Autodesk Inventor part; units mm, degrees
ref_plane "YZ Plane" through (0, 0, 0) normal (1, 0, 0) x (0, 1, 0)
ref_plane "XZ Plane" through (0, 0, 0) normal (0, 1, 0) x (-1, 0, 0)
ref_plane "XY Plane" through (0, 0, 0) normal (0, 0, 1) x (1, 0, 0)
sketch "Sketch15" plane through (0, 0, 0) normal (1, 0, 0) x (0, 1, 0)
  line L0 (0, 0) -> (50.8, 0)
  line L1 (50.8, 0) -> (50.8, 25.4)
  line L2 (50.8, 25.4) -> (0, 25.4)
  line L3 (0, 25.4) -> (0, 0)
  line L4 (48.26, 22.86) -> (2.54, 22.86)
  line L5 (2.54, 22.86) -> (2.54, 2.54)
  line L6 (2.54, 2.54) -> (48.26, 2.54)
  line L7 (48.26, 2.54) -> (48.26, 22.86)
  dimension "d46" = 25.4
  dimension "d47" = 50.8
  dimension "d48" = 2.54
  dimension "d49" = 2.54
  dimension "d50" = 2.54
  dimension "d51" = 2.54
extrude "Extrusion12" add sketch "Sketch15" along normal blind 76.2
sketch "Sketch17" plane through (0, 0, 0) normal (0, 0, -1) x (-1, 0, 0)
  line L0 (0, 2.54) -> (-76.2, 2.54)
  line L1 (0, 48.26) -> (-76.2, 48.26)
  line L2 (-73.617, 2.54) -> (-3.1161, 2.54)
  line L3 (-3.1161, 2.54) -> (-3.1161, 48.26)
  line L4 (-3.1161, 48.26) -> (-73.617, 48.26)
  line L5 (-73.617, 48.26) -> (-73.617, 2.54)
  point P0 (0, 0)
extrude "Extrusion14" add sketch "Sketch17" along normal blind 2.54
sketch "Sketch20" plane through (0, 0, 0) normal (0, 0, -1) x (-1, 0, 0)
  line L0 (0, 0) -> (25.4, 0)
  line L1 (25.4, 0) -> (0, 0)
  line L2 (0, 0) -> (0, 50.8)
  line L3 (0, 50.8) -> (25.4, 50.8)
  line L4 (25.4, 50.8) -> (25.4, 0)
  line L5 (22.86, 48.26) -> (2.54, 48.26)
  line L6 (2.54, 48.26) -> (2.54, 2.54)
  line L7 (2.54, 2.54) -> (22.86, 2.54)
  line L8 (22.86, 2.54) -> (22.86, 48.26)
  line L9 (0, 0) -> (0, 50.8)
  dimension "d71" = 25.4
  dimension "d72" = 50.8
  dimension "d73" = 2.54
  dimension "d74" = 2.54
  dimension "d75" = 2.54
  dimension "d76" = 2.54
  dimension "d78" = 0
extrude "Extrusion16" add sketch "Sketch20" against normal blind 254
sketch "Sketch21" plane through (76.2, 0, 0) normal (0, -1, 0) x (1, 0, 0)
  circle A0 centre (-38.1, 12.7) radius 2.5797
  circle A1 centre (-63.5, 12.7) radius 2.5797
  circle A2 centre (-88.9, 12.7) radius 2.5797
  circle A3 centre (-88.9, 38.1) radius 2.5797
  circle A4 centre (-88.9, 63.5) radius 2.5797
  line L0 (-76.2, 25.4) -> (0, 25.4)
  line L1 (-101.6, 0) -> (-101.6, 254)
  line L2 (-76.2, 25.4) -> (-76.2, 254)
  point P0 (-76.2, 0)
  dimension "d81" = 12.7
  dimension "d82" = 12.7
  dimension "d83" = 12.7
  dimension "d84" = 25.4
  dimension "d85" = 12.7
  dimension "d86" = 5.1594
  dimension "d87" = 5.1594
  dimension "d88" = 5.1594
  dimension "d89" = 25.4
  dimension "d90" = 25.4
  dimension "d91" = 25.4
  dimension "d92" = 5.1594
  dimension "d93" = 5.1594
  dimension "d94" = 12.7
  dimension "d95" = 12.7
extrude "Extrusion17" cut sketch "Sketch21" against normal blind 76.2
sketch "Sketch22" plane through (76.2, 50.8, 25.4) normal (0, 1, 0) x (1, 0, 0)
  circle A0 centre (-88.9, -215.9) radius 2.5797
  circle A1 centre (-88.9, -190.5) radius 2.5797
  circle A2 centre (-88.9, -165.1) radius 2.5797
  line L0 (-76.2, 0) -> (-76.2, -228.6)
  line L1 (-76.2, -228.6) -> (-101.6, -228.6)
  point P0 (-76.2, 25.4)
  dimension "d98" = 25.4
  dimension "d99" = 25.4
  dimension "d100" = 12.7
  dimension "d101" = 12.7
  dimension "d102" = 12.7
  dimension "d103" = 5.1594
  dimension "d104" = 5.1594
  dimension "d105" = 5.1594
  dimension "d108" = 12.7
extrude "Extrusion18" cut sketch "Sketch22" against normal blind 76.2
equation "\"d49\" = d48"
equation "\"d50\" = d48"
equation "\"d51\" = d48"
equation "\"d73\" = d77"
equation "\"d74\" = d77"
equation "\"d75\" = d77"
equation "\"d76\" = d77"
equation "\"d87\" = d86"
equation "\"d88\" = d86"
equation "\"d92\" = d86"
equation "\"d93\" = d86"
equation "\"d101\" = d100"
equation "\"d102\" = d100"
equation "\"d104\" = d103"
equation "\"d105\" = d103"
properties part number "left arm"
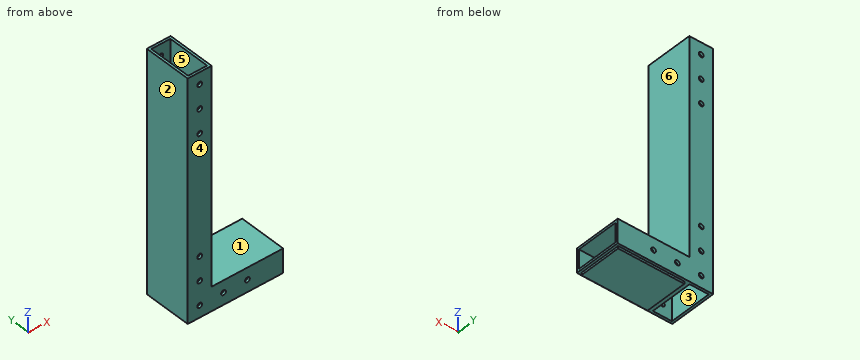
Build history of the part. All positions in model axes, mm. Face numbers are marked on the shaded views. A direction names the side the tool comes from. Give positions to 0.01 mm unless a question says otherwise; leave off trailing zeros. Order: outer loops, then holes, each group sorted by start corner. A loop starts at its lowest first (then second) coordinate and runs counter-clockwise, first axis right, second up. Notation, with made-up numbers: M -31.75,-27.5 L -23.75,-27.5 A32 cw -23.75,11.5 Z; hole C -4,-27.75 d10. An arc over 180 degrees is marked long. Put each result on its own line as item: value.
Item 1: Wall check: probe 1 along Z at (x, y) = (13, 45); probe 2 along X at (y, z) = (44, 171); probe 3 along Y at (x, z) = (-19.5, 8). Give the ranges that are in metal, low to high.
Results are:
probe 1: -2.54 to 2.54, 22.86 to 25.4
probe 2: -25.4 to -22.86, -2.54 to 0
probe 3: 0 to 2.54, 48.26 to 50.8
Item 2: Which spindle directions (+Z, -Z, +X, -X, +Y, -Y) get a long thin tool onto all of the face, cutting with end or side? Do the marked faces 1, 2 and 3. Say none if no direction does.
Results are:
face 1: +Z, +X, +Y, -Y
face 2: +Z, -Z, -X, +Y, -Y
face 3: +Z, -Z
Item 3: Cut at C-C on x = 12.7. Write the cut outline in (y, z).
Results are:
outline: M 0,0 L 2.54,0 L 2.54,-2.54 L 48.26,-2.54 L 48.26,0 L 50.8,0 L 50.8,10.12 L 48.26,10.12 L 48.26,2.54 L 2.54,2.54 L 2.54,10.12 L 0,10.12 Z; M 0,15.28 L 2.54,15.28 L 2.54,22.86 L 48.26,22.86 L 48.26,15.28 L 50.8,15.28 L 50.8,25.4 L 0,25.4 Z
Item 4: Cut at B-B on y = 26. Write the cut outline in (x, z).
Results are:
outline: M -25.4,0 L -22.86,0 L -22.86,254 L -25.4,254 Z; M -2.54,0 L 3.12,0 L 3.12,-2.54 L 73.62,-2.54 L 73.62,0 L 76.2,0 L 76.2,2.54 L 0,2.54 L 0,22.86 L 76.2,22.86 L 76.2,25.4 L 0,25.4 L 0,254 L -2.54,254 Z
Item 5: Drop flat-ended pins along their axis: pin 1 Ø6 at (y, z) = (21, 134.5) entering from +X; pin 2 Ø4 at (x, y) = (23, 27) entering from +Z; pin 3 Ø4.5 at (x, z) = (-12.7, 38.1) entering from +Y; pin 4 Ø0.8 at (y, z) = (28, -2) entering from +X. Give the stop position or say it passes through.
Results are:
pin 1: x = 0
pin 2: z = 25.4
pin 3: through
pin 4: x = 73.62
Item 6: Cut at A-A on z = 38.1. Write the cut outline in (x, y).
Results are:
outline: M -25.4,0 L -15.28,0 L -15.28,2.54 L -22.86,2.54 L -22.86,48.26 L -15.28,48.26 L -15.28,50.8 L -25.4,50.8 Z; M -10.12,0 L 0,0 L 0,50.8 L -10.12,50.8 L -10.12,48.26 L -2.54,48.26 L -2.54,2.54 L -10.12,2.54 Z
Item 7: Cut at D-D on x = 66.5. Write the cut outline in (y, z), then the cut area to 3 significant figures.
Results are:
outline: M 0,0 L 2.54,0 L 2.54,-2.54 L 48.26,-2.54 L 48.26,0 L 50.8,0 L 50.8,25.4 L 0,25.4 Z; hole M 2.54,2.54 L 48.26,2.54 L 48.26,22.86 L 2.54,22.86 Z
area: 477 mm2
Item 8: Pull direction Y, two halves, no side cores. Call the marked faces 4, 5 and 6: +Y half, -Y half, draft (parallel to the pull), parting line (faces both ways), or undercut.
Results are:
face 4: -Y half
face 5: undercut
face 6: draft
